```python
from build123d import *

# Parameters (mm, degrees)
F1_DEPTH = 19.05
F2_R     = 2.54
F3_DEPTH = 25.4
F4_R     = 5.08
F5_R     = 3.175
F6_W     = 25.4
F6_H     = 12.7
F7_DEPTH = 9.017


with BuildPart() as f1:
    # F0 (on Front) → F1 (new body)
    with BuildSketch(Plane.XZ):
        Polygon((-12.7, 0), (0, 0), (12.7, 0), (31.75, 0), (31.75, 3.175), (19.05, 3.175), (19.05, 9.525), (-19.05, 9.525), (-19.05, 3.175), (-31.75, 3.175), (-31.75, 0), align=None)
    extrude(amount=F1_DEPTH)

    # F2 (on face) → F3 (cut)
    with BuildSketch(Plane(origin=(0, 0, 0), x_dir=(1, 0, 0), z_dir=(0, 0, -1))):
        with Locations((-25.4, 9.525)):
            Circle(F2_R)
        with Locations((25.4, 9.525)):
            Circle(F2_R)
    extrude(amount=-F3_DEPTH, mode=Mode.SUBTRACT)

    # F4
    f4_edges = [f1.edges().sort_by_distance(p)[0] for p in [
        (-31.75, -19.05, 1.5875),
        (31.75, -19.05, 1.5875),
        (31.75, 0, 1.5875),
        (-31.75, 0, 1.5875),
        (19.05, 0, 6.35),
        (-19.05, 0, 6.35),
        (19.05, -19.05, 6.35),
        (-19.05, -19.05, 6.35),
    ]]
    fillet(f4_edges, radius=F4_R)

    # F5
    f5_edges = [f1.edges().sort_by_distance(p)[0] for p in [
        (-17.562102, -17.562102, 9.525),
    ]]
    fillet(f5_edges, radius=F5_R)

    # F6 (on face) → F7 (cut)
    with BuildSketch(Plane(origin=(0, 0, 0), x_dir=(1, 0, 0), z_dir=(0, 0, -1))):
        with Locations((0, 9.525)):
            Rectangle(F6_W, F6_H)
    extrude(amount=-F7_DEPTH, mode=Mode.SUBTRACT)


solid = f1.part
```
Verification items for the finished model (mm, model axes). A direction names the side the tool comes from. Round coordinates to 2 decimals unless told otherwise and drop trailing zeros. Write each loop counter-clockwise with the first axis right and the second up, starting at its lowest first coordinate (ties: lowest second). Pieces come first, ordered by that corner, then holes. Notation, with made-up numbers: (-25, 39.25) -> (6, 39.25) arc R23 ccw to (6, 73.25) -> close; hole circle Ø8 at (42.25, 36.25). An arc over 180 degrees is marked (long way). Write each question's results on one line, items separated by ' | '. Start each with the question number.
1. Cross-section at C-C (x = 5). Enter the section's corners in (y, z) (3 decimals), then the cut area to 3 significant figures.
2. Cross-section at B-B (z = 5.5). Enter the section's corners in (x, y) (3 decimals).
3. Cross-section at D-D (z = 2.25). Enter the section's corners in (x, y) (3 decimals), then the cut area to 3 significant figures.
4. Cross-section at A-A (x = 25.4). Enter the section's corners in (y, z) (3 decimals), then the cut area to 3 significant figures.
5. Material ranges on probe 1 along Y at (x, z) = (25.4, 1) (3 decimals); probe 2 along Y at (x, z) = (6, 2) (3 decimals); probe 3 along X at (y, z) = (-11.5, 0.5), recorded low to high. Write a range as from..to.
6. Depth check by flat-ended pin: P1, Ø5.5, axis at x = 23, y = -14, coming from the +Z side (3 decimals); P2, Ø5.5, axis at x = -20.5, y = -6, coming from the +Z side; P3, Ø2, axis at y = -16.5, z = 3.5, coming from the +X side. Enter the tip coordinate at first touch or a pass-through.
7. Draft check along Y on faces 4 (the flat face through (19.05, -9, 5)), 5 (the flat face through (0, -15.875, 4)), 6 (the cylindrical face through (0.196, -0.905, 8.57)). Enter one of: +Y half, -Y half, draft (parallel to the pull), parting line (faces both ways), or undercut.
8. Set-up check for faces 1 (the cylindrical face through (17.522, -17.601, 4.785)), 2 (the flat face through (-19.05, -9, 5)), 3 (the flat face through (12.7, -9, 4)): record each of +Z, -Z, +X, -X, +Y, -Y from which the full face is reachable in a straight line by a thin tool's end or side.
Solutions:
1) outline: (-19.05, 0) -> (-15.875, 0) -> (-15.875, 9.017) -> (-3.175, 9.017) -> (-3.175, 0) -> (0, 0) -> (0, 6.35) arc R3.175 ccw to (-3.175, 9.525) -> (-15.875, 9.525) arc R3.175 ccw to (-19.05, 6.35) -> close | area: 62.6 mm2
2) outline: (-19.05, -13.97) arc R5.08 ccw to (-13.97, -19.05) -> (13.97, -19.05) arc R5.08 ccw to (19.05, -13.97) -> (19.05, -5.08) arc R5.08 ccw to (13.97, 0) -> (-13.97, 0) arc R5.08 ccw to (-19.05, -5.08) -> close; hole (-12.7, -15.875) -> (12.7, -15.875) -> (12.7, -3.175) -> (-12.7, -3.175) -> close
3) outline: (-31.75, -13.97) arc R5.08 ccw to (-26.67, -19.05) -> (26.67, -19.05) arc R5.08 ccw to (31.75, -13.97) -> (31.75, -5.08) arc R5.08 ccw to (26.67, 0) -> (-26.67, 0) arc R5.08 ccw to (-31.75, -5.08) -> close; hole circle Ø5.08 at (-25.4, -9.525); hole (-12.7, -15.875) -> (12.7, -15.875) -> (12.7, -3.175) -> (-12.7, -3.175) -> close; hole circle Ø5.08 at (25.4, -9.525) | area: 824 mm2
4) outline: (-19.05, 0) -> (-12.065, 0) -> (-12.065, 3.175) -> (-19.05, 3.175) -> close; (-6.985, 0) -> (0, 0) -> (0, 3.175) -> (-6.985, 3.175) -> close | area: 44.4 mm2
5) probe 1: y = -19.05..-12.065, -6.985..0 | probe 2: y = -19.05..-15.875, -3.175..0 | probe 3: x = -31.75..-27, -23.8..-12.7, 12.7..23.8, 27..31.75
6) P1: stops at z = 3.175 | P2: stops at z = 8.91 | P3: stops at x = 31.5
7) face 4: draft | face 5: undercut | face 6: +Y half
8) face 1: +Z, +X, -Y | face 2: +Z, -X, +Y, -Y | face 3: -Z
